Model file for the job. Use its own axes, mm. A direction names the side the tool comes from. Round coordinates to 2 decimals unless told otherwise and drop trailing zeros. Order: outer loops, then holes, each group sorted by start corner. A loop starts at its lowest first (then second) coordinate and runs counter-clockwise, first axis right, second up. Notation, with made-up numbers: (75.5, 55.5) -> (89.5, 55.5) arc R19 ccw to (89.5, 86.5) -> close; hole circle Ø10 at (14.25, 8.25). An arc over 180 degrees is marked (long way). Put each result on its own line as item: value. Start each with the question number.
Q1. Flat gauge pins, fed straight in: P1, Ø5, axis at y = 6.5, z = 10.5, coming from the +X side; P2, Ø3, axis at y = 5, z = -2.5, coming from the -X side; P3, Ø1.5, axis at x = -1, z = -7.5, coming from the +Y side. Where does each tip first touch, or does it go through?
Q2. Cut at A-A, the plane y = 1.5. List the corners of the cut face in (x, z).
Q3. Cut at D-D, the plane z = -9.25. List the corners of the cut face in (x, y), and give its area (3 significant figures).
Q4. Pull direction Z, two halves, no side cores. Call faces 1 (the face through (4.05, 3, 0)), 2 (the face through (-9.52, 1.23, 0.78)), 3 (the face through (4, 6, 15)): released by +Z, released by -Z, zero draft, split by the parting line, or undercut.
Q5. Probe L1, parallel to Z at x = 12, y = 0.95; L2, parallel to X at y = 1.5, z = 5; L3, parallel to Y at x = -9, z = 12. List the from-to ranges inside material, lowest first.
Q6. Cut at C-C, the plane x = -12. List the corners of the cut face in (y, z).
Q7. Cut at B-B, the plane z = 0. List the corners of the cut face in (x, y).
Q8. 3-axis set-ups, long thin cutter, end or side, ignore diameter. For faces 4 (the face through (-4.05, 3, 0)), 5 (the face through (-9, 2.5, 0)), 6 (the face through (8, 0, 0)), 7 (the face through (14.48, 1.23, 0.78)), 8 (the face through (9, 2.5, 0)): which of +Z, -Z, +X, -X, +Y, -Y reach the whole face in a straight line?
from build123d import *

# Parameters (mm, degrees)
F1_DEPTH = 15
F2_R     = 2.6
F3_DEPTH = 10.601
F4_R     = 1


with BuildPart() as f1:
    # F0 (on Top) → F1 (new body, symmetric)
    with BuildSketch(Plane.XY):
        with BuildLine():
            Line((-4.05, 0), (-4.05, 4.05))
            ThreePointArc((-4.05, 4.05), (0, 8.1), (4.05, 4.05))
            Line((4.05, 4.05), (4.05, 0))
            Line((4.05, 0), (17, 0))
            Line((17, 0), (17, 2.5))
            Line((17, 2.5), (6.55, 2.5))
            Line((6.55, 2.5), (6.55, 4.05))
            ThreePointArc((6.55, 4.05), (0, 10.6), (-6.55, 4.05))
            Line((-6.55, 4.05), (-6.55, 2.5))
            Line((-6.55, 2.5), (-17, 2.5))
            Line((-17, 2.5), (-17, 0))
            Line((-17, 0), (-4.05, 0))
        make_face()
    extrude(amount=F1_DEPTH, both=True)

    # F2 (on face) → F3 (cut, through all)
    with BuildSketch(Plane.XZ):
        with Locations((-12, 0)):
            Circle(F2_R)
        with Locations((12, 0)):
            Circle(F2_R)
    extrude(amount=-F3_DEPTH, mode=Mode.SUBTRACT)

    # F4
    f4_edges = [f1.edges().sort_by_distance(p)[0] for p in [
        (-4.05, 0, 0),
        (4.05, 0, 0),
        (6.55, 2.5, 0),
        (-6.55, 2.5, 0),
    ]]
    fillet(f4_edges, radius=F4_R)


solid = f1.part
Ans:
1. P1: stops at x = 6.55
1. P2: stops at x = -6.55
1. P3: stops at y = 10.6
2. outline: (-17, -15) -> (-4.05, -15) -> (-4.05, 15) -> (-17, 15) -> close; (4.05, -15) -> (17, -15) -> (17, 15) -> (4.05, 15) -> close; hole circle Ø5.2 at (-12, 0); hole circle Ø5.2 at (12, 0)
3. outline: (-17, 0) -> (-5.05, 0) arc R1 ccw to (-4.05, 1) -> (-4.05, 4.05) arc R4.05 cw to (4.05, 4.05) -> (4.05, 1) arc R1 ccw to (5.05, 0) -> (17, 0) -> (17, 2.5) -> (7.55, 2.5) arc R1 cw to (6.55, 3.5) -> (6.55, 4.05) arc R6.55 ccw to (-6.55, 4.05) -> (-6.55, 3.5) arc R1 cw to (-7.55, 2.5) -> (-17, 2.5) -> close
3. area: 114 mm^2
4. face 1: zero draft
4. face 2: undercut
4. face 3: released by +Z
5. L1: z = -15 to -2.6, 2.6 to 15
5. L2: x = -17 to -4.05, 4.05 to 17
5. L3: y = 0 to 2.5
6. outline: (0, -15) -> (2.5, -15) -> (2.5, -2.6) -> (0, -2.6) -> close; (0, 2.6) -> (2.5, 2.6) -> (2.5, 15) -> (0, 15) -> close
7. outline: (-17, 0) -> (-14.6, 0) -> (-14.6, 2.5) -> (-17, 2.5) -> close; (-9.4, 0) -> (-5.05, 0) arc R1 ccw to (-4.05, 1) -> (-4.05, 4.05) arc R4.05 cw to (4.05, 4.05) -> (4.05, 1) arc R1 ccw to (5.05, 0) -> (9.4, 0) -> (9.4, 2.5) -> (7.55, 2.5) arc R1 cw to (6.55, 3.5) -> (6.55, 4.05) arc R6.55 ccw to (-6.55, 4.05) -> (-6.55, 3.5) arc R1 cw to (-7.55, 2.5) -> (-9.4, 2.5) -> close; (14.6, 0) -> (17, 0) -> (17, 2.5) -> (14.6, 2.5) -> close
8. face 4: +Z, -Z, -Y
8. face 5: +Z, -Z, -X, +Y
8. face 6: +Z, -Z, +X, -X, -Y
8. face 7: +Y, -Y
8. face 8: +Z, -Z, +X, +Y
